```python
from build123d import *

# Parameters (mm, degrees)
BOSS_EXTRUDE1_DEPTH = 3
CHAMFER1_SIZE       = 5


with BuildPart() as part:
    # Sketch1 → Boss-Extrude1 (new body)
    with BuildSketch(Plane(origin=(0, 0, 0), x_dir=(0, 0, -1), z_dir=(1, 0, 0))):
        Polygon((-60, 5), (-10, 5), (-10, 8), (0, 8), (0, 5), (30, 5), (30, 8), (40, 8), (40, 5), (90, 5), (90, -5), (-90, -5), (-90, 5), (-70, 5), (-70, 8), (-60, 8), align=None)
    extrude(amount=BOSS_EXTRUDE1_DEPTH)

    # Chamfer1
    chamfer1_edges = [part.edges().sort_by_distance(p)[0] for p in [
        (1.5, -5, 90),
    ]]
    chamfer(chamfer1_edges, length=CHAMFER1_SIZE)


solid = part.part
```
Verification items for the finished model (mm, model axes). A direction names the side the tool comes from. Give positions to 0.01 mm unless a question says otherwise; leave off trailing zeros. Order: outer loops, then holes, each group sorted by start corner. A loop starts at its lowest first (then second) coordinate and runs counter-clockwise, first axis right, second up. Notation, with made-up numbers: (51, -37.75) - (87, -37.75) arc R36 cw to (87, -2.75) - close; hole circle Ø3 at (-34, 86). An arc over 180 degrees is marked (long way). Answer as CSV lines item,"result". Start each with the question number.
Item 1: Access from +Z, -Z, +X, -X, +Y, -Y to the whole of each face (thin tool, end or side, straight path). Record for faces 1 (the face through (1, 8, 65)), 2 (the face through (1, 6, 70)), 3 (the face through (1, 7, -40)), 4 (the face through (1, 7, 60)), 5 (the face through (0, 0, -1)).
Item 2: Material ranges on L1, parallel to Z at x = 0.35, y = 5.5; L2, parallel to Y at x = 1.35, z = -72.5; L3, parallel to Z at x = 2.15, y = -0.5, recorded low to high.
Item 3: Mould release check, pull along Z, two halves, no side actions. Record for faces 6 (the face through (1, 6, -30)), 7 (the face through (1, 2, 90)), 8 (the face through (3, 0, -1)): released by +Z, released by -Z, zero draft, split by the parting line, or undercut.
Item 4: Section check A-A, the plane x = 1.65. Record the boundary of the cut face in (y, z), plus the area to 3 significant figures.
Item 5: Gauge pin test, flat ends, axial feed: pin 1 (1.5 mm diameter, centred on x = 1, y = 6.5, fed in from +Z); pin 2 (0.9 mm diameter, centred on x = 2, z = -9, fed in from +Y); pin 3 (1 mm diameter, centred on x = 1.5, y = -1.5, fed in from +Z). Record the tip position at first contact, or that the pin passes through.
Item 6: Section check B-B, the plane z = 21. Record the boundary of the cut face in (x, y).
Filled in:
1,face 1,"+Z, -Z, +X, -X, +Y"
1,face 2,"+Z, +X, -X, +Y"
1,face 3,"-Z, +X, -X, +Y"
1,face 4,"+X, -X, +Y"
1,face 5,"+Z, -Z, -X, +Y, -Y"
2,L1,"-40 to -30, 0 to 10, 60 to 70"
2,L2,"-5 to 5"
2,L3,"-90 to 89.5"
3,face 6,"undercut"
3,face 7,"released by +Z"
3,face 8,"zero draft"
4,outline,"(-5, -90) - (5, -90) - (5, -40) - (8, -40) - (8, -30) - (5, -30) - (5, 0) - (8, 0) - (8, 10) - (5, 10) - (5, 60) - (8, 60) - (8, 70) - (5, 70) - (5, 90) - (0, 90) - (-5, 85) - close"
4,area,"1,880 mm^2"
5,pin 1,"z = 70"
5,pin 2,"y = 5"
5,pin 3,"z = 89"
6,outline,"(0, -5) - (3, -5) - (3, 5) - (0, 5) - close"
